Autodesk Inventor part; units mm, degrees
ref_plane "YZ Plane" through (0, 0, 0) normal (1, 0, 0) x (0, 1, 0)
ref_plane "XZ Plane" through (0, 0, 0) normal (0, 1, 0) x (-1, 0, 0)
ref_plane "XY Plane" through (0, 0, 0) normal (0, 0, 1) x (1, 0, 0)
sketch "Sketch1" plane through (0, 0, 0) normal (0, 1, 0) x (-1, 0, 0)
  line L0 (12.5, 12.5) -> (-12.5, 12.5)
  line L1 (-12.5, 12.5) -> (-12.5, -12.5)
  line L2 (-12.5, -12.5) -> (12.5, -12.5)
  line L3 (12.5, -12.5) -> (12.5, 12.5)
  line L4 (57.15, 6) -> (31.15, 6)
  line L5 (31.15, 6) -> (31.15, -6)
  line L6 (31.15, -6) -> (57.15, -6)
  line L7 (57.15, -6) -> (57.15, 6)
  line L8 (-31.15, 6) -> (-57.15, 6)
  line L9 (-57.15, 6) -> (-57.15, -6)
  line L10 (-57.15, -6) -> (-31.15, -6)
  line L11 (-31.15, -6) -> (-31.15, 6)
  line L12 (9.55, 55.15) -> (-9.55, 55.15)
  line L13 (-9.55, 55.15) -> (-9.55, 36.05)
  line L14 (-9.55, 36.05) -> (9.55, 36.05)
  line L15 (9.55, 36.05) -> (9.55, 55.15)
  line L16 (9.55, -36.05) -> (-9.55, -36.05)
  line L17 (-9.55, -36.05) -> (-9.55, -55.15)
  line L18 (-9.55, -55.15) -> (9.55, -55.15)
  line L19 (9.55, -55.15) -> (9.55, -36.05)
  line L20 (57.15, 57.15) -> (-57.15, 57.15)
  line L21 (-57.15, 57.15) -> (-57.15, -57.15)
  line L22 (-57.15, -57.15) -> (57.15, -57.15)
  line L23 (57.15, -57.15) -> (57.15, 57.15)
  circle A0 centre (-28.575, -28.575) radius 16.0636
  line L24 (-28.575, -28.575) -> (-44.6386, -28.575)
  line L25 (-28.575, -28.575) -> (-20.5432, -42.4865)
  line L26 (-28.575, -28.575) -> (-12.5114, -28.575) construction
  line L27 (-28.575, -28.575) -> (-20.5432, -14.6635)
  circle A1 centre (-24.5591, -21.6193) radius 3.2
  circle A2 centre (-24.5591, -35.5307) radius 3.2
  circle A3 centre (-36.6068, -28.575) radius 3.2
  line L28 (0, 0) -> (-12.5, -12.5)
  circle A4 centre (-28.575, 28.575) radius 16.0636
  line L29 (-28.575, 28.575) -> (-44.6386, 28.575)
  line L30 (-28.575, 28.575) -> (-20.5432, 14.6635)
  line L31 (-28.575, 28.575) -> (-20.5432, 42.4865)
  circle A5 centre (-24.5591, 35.5307) radius 3.2
  circle A6 centre (-24.5591, 21.6193) radius 3.2
  circle A7 centre (-36.6068, 28.575) radius 3.2
  circle A8 centre (28.575, 28.575) radius 16.0636
  line L32 (28.575, 28.575) -> (12.5114, 28.575)
  line L33 (28.575, 28.575) -> (36.6068, 14.6635)
  line L34 (28.575, 28.575) -> (36.6068, 42.4865)
  circle A9 centre (32.5909, 35.5307) radius 3.2
  circle A10 centre (32.5909, 21.6193) radius 3.2
  circle A11 centre (20.5432, 28.575) radius 3.2
  circle A12 centre (28.575, -28.575) radius 16.0636
  line L35 (28.575, -28.575) -> (12.5114, -28.575)
  line L36 (28.575, -28.575) -> (36.6068, -42.4865)
  line L37 (28.575, -28.575) -> (36.6068, -14.6635)
  circle A13 centre (32.5909, -21.6193) radius 3.2
  circle A14 centre (32.5909, -35.5307) radius 3.2
  circle A15 centre (20.5432, -28.575) radius 3.2
  line L38 (34.1909, 38.302) -> (36.6068, 42.4865)
  line L39 (30.9909, 32.7595) -> (28.575, 28.575)
  line L40 (30.9909, 24.3905) -> (28.575, 28.575)
  line L41 (34.1909, 18.848) -> (36.6068, 14.6635)
  line L42 (23.7432, 28.575) -> (28.575, 28.575)
  line L43 (17.3432, 28.575) -> (12.5114, 28.575)
  line L44 (28.575, 28.575) -> (23.7432, 28.575)
  line L45 (-28.575, 28.575) -> (-26.1591, 24.3905)
  line L46 (-22.9591, 18.848) -> (-20.5432, 14.6635)
  line L47 (-26.1591, 32.7595) -> (-28.575, 28.575)
  line L48 (-22.9591, 38.302) -> (-20.5432, 42.4865)
  line L49 (-39.8068, 28.575) -> (-44.6386, 28.575)
  line L50 (-33.4068, 28.575) -> (-28.575, 28.575)
  line L51 (-22.9591, 18.848) -> (-20.5432, 14.6635)
  line L52 (-44.6386, -28.575) -> (-39.8068, -28.575)
  line L53 (-33.4068, -28.575) -> (-28.575, -28.575)
  line L54 (-28.575, -28.575) -> (-26.1591, -32.7595)
  line L55 (-22.9591, -38.302) -> (-20.5432, -42.4865)
  line L56 (-28.575, -28.575) -> (-26.1591, -24.3905)
  line L57 (-22.9591, -18.848) -> (-20.5432, -14.6635)
  line L58 (0, 0) -> (0, -57.15)
  line L59 (0, 0) -> (-57.15, 0)
  line L60 (0, 0) -> (-31.15, 0)
  line L61 (0, 0) -> (0, -36.05)
  line L62 (0, 0) -> (0, -12.5)
  line L63 (0, 0) -> (-12.5, 0)
  line L64 (-57.15, 0) -> (-57.15, -6)
  line L65 (-57.15, 0) -> (-57.15, -57.15)
  line L66 (-57.15, -57.15) -> (0, -57.15)
  line L67 (0, -55.15) -> (0, -57.15)
  line L68 (0, -36.05) -> (0, -55.15)
  line L69 (0, -36.05) -> (0, -12.5)
  point P0 (-28.575, 28.575)
  point P1 (28.575, 28.575)
  point P2 (28.575, -28.575)
  dimension "d2" = 25
  dimension "d3" = 25
  dimension "d4" = 12.5
  dimension "d5" = 12.5
  dimension "d6" = 6
  dimension "d7" = 12
  dimension "d8" = 26
  dimension "d9" = 26
  dimension "d10" = 6
  dimension "d11" = 12
  dimension "d12" = 19.1
  dimension "d13" = 19.1
  dimension "d14" = 9.55
  dimension "d15" = 19.1
  dimension "d16" = 19.1
  dimension "d17" = 9.55
  dimension "d22" = 0
  dimension "d23" = 0
  dimension "d24" = 2
  dimension "d25" = 2
  dimension "d26" = 114.3
  dimension "d28" = 57.15
  dimension "d29" = 57.15
  dimension "d30" = 114.3
  dimension "d37" = 28.575
  dimension "d38" = 28.575
  dimension "d39" = 6.4
  dimension "d40" = 6.4
  dimension "d41" = 6.4
  dimension "d43" = 120
  dimension "d44" = 120
  dimension "d45" = 32.1272
  dimension "d46" = 28.575
  dimension "d47" = 28.575
  dimension "d48" = 28.575
  dimension "d49" = 28.575
  dimension "d50" = 28.575
  dimension "d51" = 28.575
  dimension "d52" = 6.4
  dimension "d53" = 6.4
  dimension "d54" = 6.4
  dimension "d55" = 120
  dimension "d56" = 120
  dimension "d57" = 32.1272
  dimension "d58" = 6.4
  dimension "d59" = 6.4
  dimension "d60" = 6.4
  dimension "d61" = 120
  dimension "d62" = 120
  dimension "d63" = 32.1272
  dimension "d64" = 6.4
  dimension "d65" = 6.4
  dimension "d66" = 6.4
  dimension "d67" = 120
  dimension "d68" = 120
  dimension "d69" = 32.1272
extrude "Extrusion1" add sketch "Sketch1" along normal blind 7 contours L1 L2 L58 L16 L17 L18 L22 L21 L10 L11 L59 | A0 L25 A2 L27 A1 | L27 A1 L24 A3 A0 | A0 L24 A3 L25 A2
sketch "Sketch2" plane through (0, 0, 0) normal (0, -1, 0) x (1, 0, 0)
  circle A0 centre (36.6068, -28.575) radius 3.2
  circle A1 centre (36.6068, -28.575) radius 3.2
  circle A2 centre (24.5591, -21.6193) radius 3.2
  circle A3 centre (24.5591, -21.6193) radius 3.2
  circle A4 centre (24.5591, -35.5307) radius 3.2
  circle A5 centre (24.5591, -35.5307) radius 3.2
  point P0 (0, 0)
extrude "Extrusion2" add sketch "Sketch2" against normal blind 2
sketch "Sketch3" plane through (0, 0, 0) normal (0, -1, 0) x (1, 0, 0)
  line L0 (31.15, -6) -> (57.15, -6)
  line L1 (57.15, -6) -> (57.15, 0)
  line L2 (57.15, 0) -> (31.15, 0)
  line L3 (31.15, 0) -> (31.15, -6)
  point P0 (0, 0)
extrude "Extrusion3" add sketch "Sketch3" against normal blind 4.65
sketch "Sketch4" plane through (0, 7, 0) normal (0, 1, 0) x (1, 0, 0)
  line L0 (9.55, 55.15) -> (0, 55.15)
  line L1 (0, 55.15) -> (0, 36.05)
  line L2 (0, 36.05) -> (9.55, 36.05)
  line L3 (9.55, 36.05) -> (9.55, 55.15)
  point P0 (0, 0)
extrude "Extrusion4" add sketch "Sketch4" against normal blind 2.84
mirror "Mirror1" about plane through (0, 0, -36.05) normal (-1, 0, 0)
mirror "Mirror2" about plane through (-12.5, 0, 0) normal (0, 0, 1)
properties part number "Prototype1"
Can you work these out from the model? Positions are in its coordinate system, mm. A direction names the side the tool comes from. Coordinates: 2 decimals unless noted, no trailing zeros. Loops run counter-clockwise (first coordinate to the right, second up) from the corner with the lowest first, then second, coordinate; pieces in that order, holes last.
1) I need wall thicknesses on probe 1 along Z at (x, y) = (-42.5, 6.75); probe 2 along X at (y, z) = (2, 5); probe 3 along Z at (x, y) = (27, 5.25). Which ranges of each line are inside material? Lowest first, please.
2) Imagine slicing it at C-C on z = 2. List the corners of the cut face in (x, y) for me.
3) Imagine slicing it at D-D on x = -47.5. List the corners of the cut face in (y, z) for me.
4) Thinking about a two-plate mould opening in Z: for faces 1 (the flat face through (-25, 2, -22)), 2 (the flat face through (57.15, 3, -1)), which applies, pulls with the +Z half, pulls with the -Z half, needs draft (parallel to the pull), parting line crosses it, or undercut?
5) Imagine slicing it at A-A on z = -10. List the corners of the cut face in (x, y) for me, plus the area to 3 significant figures.
6) Which directions (+Z, -Z, +X, -X, +Y, -Y) give clear straight access to the entire face, cutting with the end or side of a thin tool? Please do faces 3 (the flat face through (-44, 4.65, 0)), 4 (the cylindrical face through (-25, 4.5, 38.7)), 5 (the flat face through (0, 4.16, -46)), 6 (the flat face through (-1, 7, -14)), 7 (the flat face through (12.5, 3, 0)).
7) For pin 1 (1.9 mm diameter, centred on x = 26, z = -34, fed in from +Y), with a flat end and sliding along its axis, tell me the tip position at first contact or that it passes through.
8) Imagine slicing it at B-B on x = -6.5. List the corners of the cut face in (y, z) for me, plus the area to 3 significant figures.
Completed:
1. probe 1: z = -57.15 to -6, 6 to 57.15
1. probe 2: x = -57.15 to -12.5, 12.5 to 57.15
1. probe 3: z = -57.15 to -37.6, -33.46 to -23.69, -19.55 to 19.55, 23.69 to 33.46, 37.6 to 57.15
2. outline: (-57.15, 0) - (-12.5, 0) - (-12.5, 7) - (-31.15, 7) - (-31.15, 4.65) - (-57.15, 4.65) - close; (12.5, 0) - (57.15, 0) - (57.15, 4.65) - (31.15, 4.65) - (31.15, 7) - (12.5, 7) - close
3. outline: (0, -57.15) - (7, -57.15) - (7, -6) - (4.65, -6) - (4.65, 6) - (7, 6) - (7, 57.15) - (0, 57.15) - close
4. face 1: undercut
4. face 2: needs draft
5. outline: (-57.15, 0) - (-12.5, 0) - (-12.5, 7) - (-57.15, 7) - close; (12.5, 0) - (57.15, 0) - (57.15, 7) - (12.5, 7) - close
5. area: 625 mm2
6. face 3: -X, +Y
6. face 4: +Y
6. face 5: -Y
6. face 6: +Z, -Z, +X, -X, +Y
6. face 7: +Y, -Y
7. pin 1: stops at y = 2
8. outline: (0, -57.15) - (7, -57.15) - (7, -12.5) - (0, -12.5) - (0, -36.05) - (4.16, -36.05) - (4.16, -55.15) - (0, -55.15) - close; (0, 12.5) - (7, 12.5) - (7, 57.15) - (0, 57.15) - (0, 55.15) - (4.16, 55.15) - (4.16, 36.05) - (0, 36.05) - close
8. area: 466 mm2
